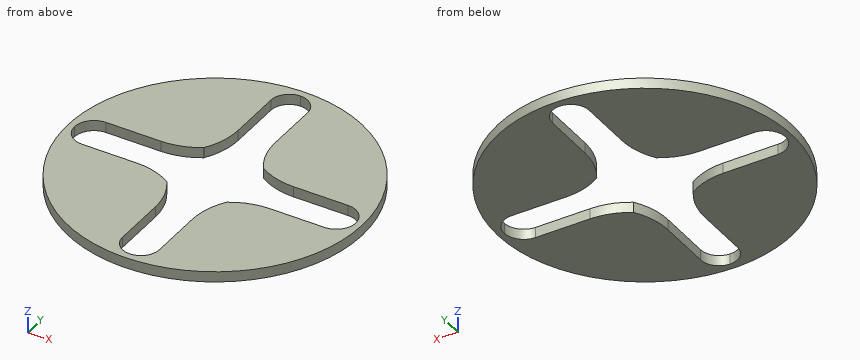
```python
from build123d import *

# Parameters (mm, degrees)
F0_R        = 44.45
F0_R_2      = 12.7
F1_DEPTH    = 3.175
F3_DEPTH    = 25.4
F4_T1_DEPTH = 48.6343800889
F4_T3_DEPTH = 47.4571451006
F4_T5_DEPTH = 47.1924378771


# Not quite as in the source:
# - a fillet or chamfer that OpenCascade refuses, or shapes differently, is made with other operations: its cross-section is extruded or revolved along the edge and cut away or added


with BuildPart() as f1:
    # F0 (on Top) → F1 (new body)
    with BuildSketch(Plane.XY):
        Circle(F0_R)
        Circle(F0_R_2, mode=Mode.SUBTRACT)
    extrude(amount=F1_DEPTH)

    # F2 (on face) → F3 (cut)
    with BuildSketch(Plane.XY.offset(3.175)):
        with BuildLine():
            Line((-42.5250590142, 0), (-12.7, 0))
            ThreePointArc((-12.7, 0), (-12.3276162196, 3.0528475792), (-11.2323026233, 5.9266666667))
            Line((-11.2323026233, 5.9266666667), (-36.6323026233, 5.9266666667))
            ThreePointArc((-36.6323026233, 5.9266666667), (-40.8111169187, 4.1887178728), (-42.5250590142, 0))
        make_face()
        with BuildLine():
            ThreePointArc((-11.2677815117, -5.8589333333), (-12.3367504878, -3.0157233628), (-12.7, 0))
            Line((-12.7, 0), (-42.5250590142, 0))
            ThreePointArc((-42.5250590142, 0), (-40.79976808, -4.1324743979), (-36.6677815117, -5.8589333333))
            Line((-36.6677815117, -5.8589333333), (-11.2677815117, -5.8589333333))
        make_face()
        with BuildLine():
            Line((0, 12.7), (0, 42.3763238149))
            ThreePointArc((0, 42.3763238149), (-3.928862053, 40.7489358679), (-5.55625, 36.8200738149))
            Line((-5.55625, 36.8200738149), (-5.55625, 11.4200738149))
            ThreePointArc((-5.55625, 11.4200738149), (-2.8508825433, 12.3758825433), (0, 12.7))
        make_face()
        with BuildLine():
            ThreePointArc((5.55625, 36.8200738149), (3.928862053, 40.7489358679), (0, 42.3763238149))
            Line((0, 42.3763238149), (0, 12.7))
            ThreePointArc((0, 12.7), (2.8508825433, 12.3758825433), (5.55625, 11.4200738149))
            Line((5.55625, 11.4200738149), (5.55625, 36.8200738149))
        make_face()
        with BuildLine():
            ThreePointArc((5.55625, -11.4200738149), (2.8508825433, -12.3758825433), (0, -12.7))
            Line((0, -12.7), (0, -42.3763238149))
            ThreePointArc((0, -42.3763238149), (3.928862053, -40.7489358679), (5.55625, -36.8200738149))
            Line((5.55625, -36.8200738149), (5.55625, -11.4200738149))
        make_face()
        with BuildLine():
            Line((0, -42.3763238149), (0, -12.7))
            ThreePointArc((0, -12.7), (-2.8508825433, -12.3758825433), (-5.55625, -11.4200738149))
            Line((-5.55625, -11.4200738149), (-5.55625, -36.8200738149))
            ThreePointArc((-5.55625, -36.8200738149), (-3.928862053, -40.7489358679), (0, -42.3763238149))
        make_face()
        with BuildLine():
            ThreePointArc((11.2323026233, 5.9266666667), (12.3276162196, 3.0528475792), (12.7, 0))
            Line((12.7, 0), (42.5250590142, 0))
            ThreePointArc((42.5250590142, 0), (40.8111169187, 4.1887178728), (36.6323026233, 5.9266666667))
            Line((36.6323026233, 5.9266666667), (11.2323026233, 5.9266666667))
        make_face()
        with BuildLine():
            Line((42.5250590142, 0), (12.7, 0))
            ThreePointArc((12.7, 0), (12.3367504878, -3.0157233628), (11.2677815117, -5.8589333333))
            Line((11.2677815117, -5.8589333333), (36.6677815117, -5.8589333333))
            ThreePointArc((36.6677815117, -5.8589333333), (40.79976808, -4.1324743979), (42.5250590142, 0))
        make_face()
    extrude(amount=-F3_DEPTH, mode=Mode.SUBTRACT)

    # F4: fillet of radius 20.32 on 8 edges, made by hand

    # F4_s2 → F4_t1 (cut)
    with BuildSketch(Plane.XY.offset(-22.7296900444)):
        with BuildLine():
            ThreePointArc((-9.9524038462, -7.8892114741), (-6.6867352348, -13.8287677255), (-5.55625, -20.5119498327))
            Line((-5.55625, -20.5119498327), (-5.55625, -11.4200738149))
            ThreePointArc((-5.55625, -11.4200738149), (-7.9527563302, -9.901700195), (-9.9524038462, -7.8892114741))
        make_face()
        with BuildLine():
            ThreePointArc((9.9524038462, 7.8892114741), (6.6867352348, 13.8287677255), (5.55625, 20.5119498327))
            Line((5.55625, 20.5119498327), (5.55625, 11.4200738149))
            ThreePointArc((5.55625, 11.4200738149), (7.9527563302, 9.901700195), (9.9524038462, 7.8892114741))
        make_face()
        with BuildLine():
            ThreePointArc((-5.55625, 20.5119498327), (-6.6867352348, 13.8287677255), (-9.9524038462, 7.8892114741))
            ThreePointArc((-9.9524038462, 7.8892114741), (-7.9527563302, 9.901700195), (-5.55625, 11.4200738149))
            Line((-5.55625, 11.4200738149), (-5.55625, 20.5119498327))
        make_face()
        with BuildLine():
            ThreePointArc((5.55625, -20.5119498327), (6.6867352348, -13.8287677255), (9.9524038462, -7.8892114741))
            ThreePointArc((9.9524038462, -7.8892114741), (7.9527563302, -9.901700195), (5.55625, -11.4200738149))
            Line((5.55625, -11.4200738149), (5.55625, -20.5119498327))
        make_face()
    extrude(amount=F4_T1_DEPTH, mode=Mode.SUBTRACT)

    # F4_s4 → F4_t3 (cut)
    with BuildSketch(Plane.XY.offset(-22.1410725503)):
        with BuildLine():
            ThreePointArc((-20.1242105318, -5.8589333333), (-13.5841452612, -6.9401717761), (-7.7400809738, -10.0688205128))
            ThreePointArc((-7.7400809738, -10.0688205128), (-9.7342435034, -8.1568684811), (-11.2677815117, -5.8589333333))
            Line((-11.2677815117, -5.8589333333), (-20.1242105318, -5.8589333333))
        make_face()
        with BuildLine():
            ThreePointArc((7.7400809738, -10.0688205128), (13.5841452612, -6.9401717761), (20.1242105318, -5.8589333333))
            Line((20.1242105318, -5.8589333333), (11.2677815117, -5.8589333333))
            ThreePointArc((11.2677815117, -5.8589333333), (9.7342435034, -8.1568684811), (7.7400809738, -10.0688205128))
        make_face()
    extrude(amount=F4_T3_DEPTH, mode=Mode.SUBTRACT)

    # F4_s6 → F4_t5 (cut)
    with BuildSketch(Plane.XY.offset(-22.0087189386)):
        with BuildLine():
            ThreePointArc((7.7060731534, 10.0948717949), (13.5281820281, 6.9969020993), (20.0357901988, 5.9266666667))
            Line((20.0357901988, 5.9266666667), (11.2323026233, 5.9266666667))
            ThreePointArc((11.2323026233, 5.9266666667), (9.6958239858, 8.2024994506), (7.7060731534, 10.0948717949))
        make_face()
        with BuildLine():
            ThreePointArc((-7.7060731534, 10.0948717949), (-13.5281820281, 6.9969020993), (-20.0357901988, 5.9266666667))
            Line((-20.0357901988, 5.9266666667), (-11.2323026233, 5.9266666667))
            ThreePointArc((-11.2323026233, 5.9266666667), (-9.6958239858, 8.2024994506), (-7.7060731534, 10.0948717949))
        make_face()
    extrude(amount=F4_T5_DEPTH, mode=Mode.SUBTRACT)


solid = f1.part
```
Verification items for the finished model (mm, model axes). Coordinates: 2 decimals unless noted, no trailing zeros. Write each loop counter-clockwise with the first axis right and the second up, starting at its lowest first coordinate (ties: lowest second). Pieces come first, ordered by that corner, then holes. Notation, with made-up numbers: M 67.5,77 L 72.5,77 A20 cw 72.5,101 Z; hole C 52.25,56.25 d11. An arc over 180 degrees is marked long. Answer as a JSON object with one key per item and string values. Group by question number.
(1) Cross-section at C-C, the plane y = 17. Record the cut outline in (x, z) (3 decimals).
(2) Cross-section at B-B, the plane x = -16.5. Record the cut outline in (y, z) (3 decimals).
(3) Gauge pin test, flat ends, axial feed: pin 1 (1.6 mm diameter, centred on x = 25.5, z = 2, fed in from +Y); pin 2 (1.6 mm diameter, centred on y = 27, z = 2, fed in from +X); pin 3 (1.6 mm diameter, centred on y = -26, z = 2, fed in from +X). Record the tip position at first contact, or that the pin passes through.
(4) Cross-section at A-A, the plane z = 1.85. Record the cut outline in (x, y), and give its area (3 significant figures).
(5) Material ranges on line 1 (Y direction, x = 8, z = 1.1); line 2 (X direction, y = 14, z = 2.85); line 3 (Y direction, x = 0.5, z = 1.8), recorded low to high.
Reply:
{
 "1": {"outline": "M -41.071,0 L -5.862,0 L -5.862,3.175 L -41.071,3.175 Z; M 5.862,0 L 41.071,0 L 41.071,3.175 L 5.862,3.175 Z"},
 "2": {"outline": "M -41.274,0 L -6.185,0 L -6.185,3.175 L -41.274,3.175 Z; M 6.237,0 L 41.274,0 L 41.274,3.175 L 6.237,3.175 Z"},
 "3": {"pin 1": "y = 36.96", "pin 2": "x = 35.91", "pin 3": "x = 36.62"},
 "4": {"outline": "C 0,0 d88.9; hole M -36.67,-5.86 L -20.12,-5.86 A20.32 cw -9.02,-9.16 A20.32 cw -5.56,-20.51 L -5.56,-36.82 A5.56 ccw 5.56,-36.82 L 5.56,-20.51 A20.32 cw 9.02,-9.16 A20.32 cw 20.12,-5.86 L 36.67,-5.86 A5.89 ccw 36.63,5.93 L 20.04,5.93 A20.32 cw 9.01,9.18 A20.32 cw 5.56,20.51 L 5.56,36.82 A5.56 ccw -5.56,36.82 L -5.56,20.51 A20.32 cw -9.01,9.18 A20.32 cw -20.04,5.93 L -36.63,5.93 A5.89 ccw Z", "area": "4,310 mm²"},
 "5": {"line 1": "-43.72 to -10.85, 10.85 to 43.72", "line 2": "-42.19 to -6.63, 6.63 to 42.19", "line 3": "-44.45 to -42.35, 42.35 to 44.45"}
}
